Source: CAD feature listing. Evaluate the final solid. Frame: model axes, mm. Face numbers are marked on the shaded views. A direction names the side the tool comes from. Round coordinates to 2 decimals unless told otherwise and drop trailing zeros. Order: outer loops, then holes, each group sorted by start corner. A loop starts at its lowest first (then second) coordinate and runs counter-clockwise, first axis right, second up. Notation, with made-up numbers: (14.5, -14.75) - (37.5, -14.75) arc R24 cw to (37.5, 12.25) - close; hole circle Ø6 at (88.5, 37.25). An arc over 180 degrees is marked (long way). Use one line per item in the form item = value. Start each with the question number.
Q1. Pin query (flat end, axial travel): pin 1 Ø12.5 at (y, z) = (-50, 37.5) entering from -X; pin 2 Ø12.5 at (x, z) = (-46, 31.5) entering from +Y; pin 3 Ø5 at (x, z) = (9, 10.5) entering from +Y; pin 4 Ø1.5 at (y, z) = (-41.5, 82) entering from -X. Return the tip coordinate at first contact, or that it passes through.
Q2. Cut plane A-A, the plane x = 0. Return the cut outline in (y, z).
Q3. Draft query along Y for the marked faces 1, 2, 3 and 4. Return one class per face: released by +Y, released by -Y, zero draft, split by the parting line, or undercut.
Q4. Ray query, line 1 (Z direction, x = -26, y = 43); line 2 (X direction, y = 14, z = 33.5); line 3 (X direction, y = -23, z = 27). Return the intervals inside material, ascending. Write a range as [from, to].
Q5. Cut plane D-D, the plane y = 17. Return the cut outline in (x, z), and give its area (3 significant figures).
Q6. Set-up query: the marked faces 5, 6, 7, 8 and 9. Return all of +Z, -Z, +X, -X, +Y, -Y with unobstructed straight access to the full face (end or side cutting, diameter ignored); none if empty.
from build123d import *

# Parameters (mm, degrees)
F0_R            = 63.5
F1_DEPTH        = 12.7
F2_R            = 31.75
F3_DEPTH        = 88.9
F7_DEPTH        = 88.9010001
F8_R            = 6.35
F9_DEPTH        = 12.701
F9_COPIES_COUNT = 4
F10_R           = 25.4
F11_DEPTH       = 101.601


# Not quite as in the source:
# - a pattern or mirror of a feature is missing from the dataset's text; its kind, count and spacing are read off the source's solid


with BuildPart() as f1:
    # F0 (on Top) → F1 (new body)
    with BuildSketch(Plane.XY):
        Circle(F0_R)
    extrude(amount=F1_DEPTH)

    # F2 (on face) → F3 (join)
    with BuildSketch(Plane.XY.offset(12.7)):
        Circle(F2_R)
    extrude(amount=F3_DEPTH)

    # F4 (on Right) → F5 (revolve)
    with BuildSketch(Plane.YZ):
        Polygon((-31.75, 12.7), (-31.75, 101.6), (-63.5, 12.7), align=None)
    revolve(axis=Axis((0, 0, 73.5445022583), (0, 0, 1)))

    # F6 (on face) → F7 (cut, through all)
    with BuildSketch(Plane.XY.offset(12.7)):
        with BuildLine():
            ThreePointArc((-14.1111111111, 61.9122487333), (-44.9012806053, 44.9012806053), (-61.9122487333, 14.1111111111))
            ThreePointArc((-61.9122487333, 14.1111111111), (-60.6850472058, 8.7400792657), (-55.7210238599, 6.35))
            Line((-55.7210238599, 6.35), (-40.1609262841, 6.35))
            ThreePointArc((-40.1609262841, 6.35), (-33.3724907396, 8.3165409649), (-28.6863759172, 13.6071428571))
            ThreePointArc((-28.6863759172, 13.6071428571), (-22.4506403027, 22.4506403027), (-13.6071428571, 28.6863759172))
            ThreePointArc((-13.6071428571, 28.6863759172), (-8.3165409649, 33.3724907396), (-6.35, 40.1609262841))
            Line((-6.35, 40.1609262841), (-6.35, 55.7210238599))
            ThreePointArc((-6.35, 55.7210238599), (-8.7400792657, 60.6850472058), (-14.1111111111, 61.9122487333))
        make_face()
        with BuildLine():
            Line((-40.1609262841, -6.35), (-55.7210238599, -6.35))
            ThreePointArc((-55.7210238599, -6.35), (-60.6850472058, -8.7400792657), (-61.9122487333, -14.1111111111))
            ThreePointArc((-61.9122487333, -14.1111111111), (-44.9012806053, -44.9012806053), (-14.1111111111, -61.9122487333))
            ThreePointArc((-14.1111111111, -61.9122487333), (-8.7400792657, -60.6850472058), (-6.35, -55.7210238599))
            Line((-6.35, -55.7210238599), (-6.35, -40.1609262841))
            ThreePointArc((-6.35, -40.1609262841), (-8.3165409649, -33.3724907396), (-13.6071428571, -28.6863759172))
            ThreePointArc((-13.6071428571, -28.6863759172), (-22.4506403027, -22.4506403027), (-28.6863759172, -13.6071428571))
            ThreePointArc((-28.6863759172, -13.6071428571), (-33.3724907396, -8.3165409649), (-40.1609262841, -6.35))
        make_face()
        with BuildLine():
            Line((6.35, -40.1609262841), (6.35, -55.7210238599))
            ThreePointArc((6.35, -55.7210238599), (8.7400792657, -60.6850472058), (14.1111111111, -61.9122487333))
            ThreePointArc((14.1111111111, -61.9122487333), (44.9012806053, -44.9012806053), (61.9122487333, -14.1111111111))
            ThreePointArc((61.9122487333, -14.1111111111), (60.6850472058, -8.7400792657), (55.7210238599, -6.35))
            Line((55.7210238599, -6.35), (40.1609262841, -6.35))
            ThreePointArc((40.1609262841, -6.35), (33.3724907396, -8.3165409649), (28.6863759172, -13.6071428571))
            ThreePointArc((28.6863759172, -13.6071428571), (22.4506403027, -22.4506403027), (13.6071428571, -28.6863759172))
            ThreePointArc((13.6071428571, -28.6863759172), (8.3165409649, -33.3724907396), (6.35, -40.1609262841))
        make_face()
        with BuildLine():
            Line((40.1609262841, 6.35), (55.7210238599, 6.35))
            ThreePointArc((55.7210238599, 6.35), (60.6850472058, 8.7400792657), (61.9122487333, 14.1111111111))
            ThreePointArc((61.9122487333, 14.1111111111), (44.9012806053, 44.9012806053), (14.1111111111, 61.9122487333))
            ThreePointArc((14.1111111111, 61.9122487333), (8.7400792657, 60.6850472058), (6.35, 55.7210238599))
            Line((6.35, 55.7210238599), (6.35, 40.1609262841))
            ThreePointArc((6.35, 40.1609262841), (8.3165409649, 33.3724907396), (13.6071428571, 28.6863759172))
            ThreePointArc((13.6071428571, 28.6863759172), (22.4506403027, 22.4506403027), (28.6863759172, 13.6071428571))
            ThreePointArc((28.6863759172, 13.6071428571), (33.3724907396, 8.3165409649), (40.1609262841, 6.35))
        make_face()
    extrude(amount=F7_DEPTH, mode=Mode.SUBTRACT)

    # F8 (on face) → F9 (cut, through all)
    with BuildSketch(Plane.XY.offset(12.7)):
        with Locations((-33.675960454, 33.675960454)):
            Circle(F8_R)
    f9 = extrude(amount=-F9_DEPTH, mode=Mode.SUBTRACT)

    # F9_copies: F9 ×4 about axis
    f9_copies_axis = Axis((0, 0, 0), (0, 0, 1))
    for i in range(1, F9_COPIES_COUNT):
        add(f9.rotate(f9_copies_axis, i * 360 / F9_COPIES_COUNT), mode=Mode.SUBTRACT)

    # F10 (on face) → F11 (cut, through all)
    with BuildSketch(Plane.XY.offset(101.6)):
        Circle(F10_R)
    extrude(amount=-F11_DEPTH, mode=Mode.SUBTRACT)


solid = f1.part
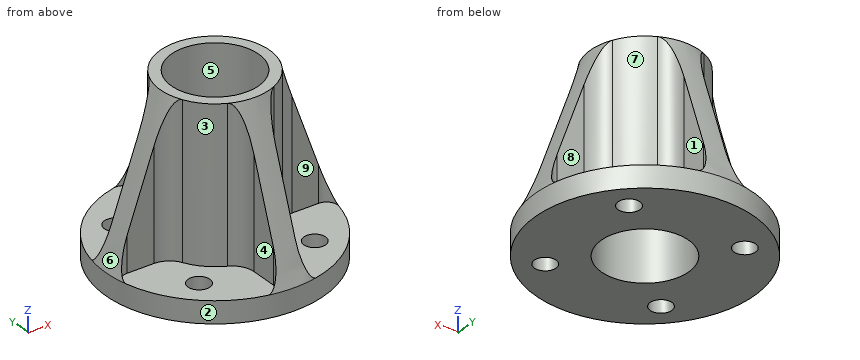
Completed:
q1.pin_1 = -6.35
q1.pin_2 = 6.36
q1.pin_3 = 63.17
q1.pin_4 = through
q2.outline = (-63.5, 0) - (-25.4, 0) - (-25.4, 101.6) - (-31.75, 101.6) - (-63.5, 12.7) - close; (25.4, 0) - (63.5, 0) - (63.5, 12.7) - (31.75, 101.6) - (25.4, 101.6) - close
q3.face_1 = undercut
q3.face_2 = split by the parting line
q3.face_3 = released by -Y
q3.face_4 = undercut
q4.line_1 = [0, 12.7]
q4.line_2 = [-28.5, -21.19], [21.19, 28.5]
q4.line_3 = [-21.89, -10.78], [10.78, 21.89]
q5.outline = (-61.18, 0) - (-18.87, 0) - (-18.87, 101.6) - (-26.82, 101.6) - (-26.82, 12.7) - (-61.18, 12.7) - close; (18.87, 0) - (61.18, 0) - (61.18, 12.7) - (26.82, 12.7) - (26.82, 101.6) - (18.87, 101.6) - close
q5.area = 2,490 mm2
q6.face_5 = +Z, -Z
q6.face_6 = +Z, -X
q6.face_7 = +Z, +X, +Y
q6.face_8 = +Z, +Y
q6.face_9 = +Z, -Y
